Input: part model. Units: mm. Frame: model coordinates. Face numbers are marked on the shaded views. Round coordinates to 2 decimals unless told otherwise and drop trailing zeros. Order: outer loops, then holes, each group sorted by start corner. A loop starts at its lowest first (then second) coordinate and runs counter-clockwise, first axis right, second up. Notation, with made-up numbers: (81, 42) -> (128, 42) arc R12 cw to (128, 61) -> close; hole circle Ø10 at (38, -6.5). An arc over 180 degrees is marked (long way). Use a Markdown table: item, result.
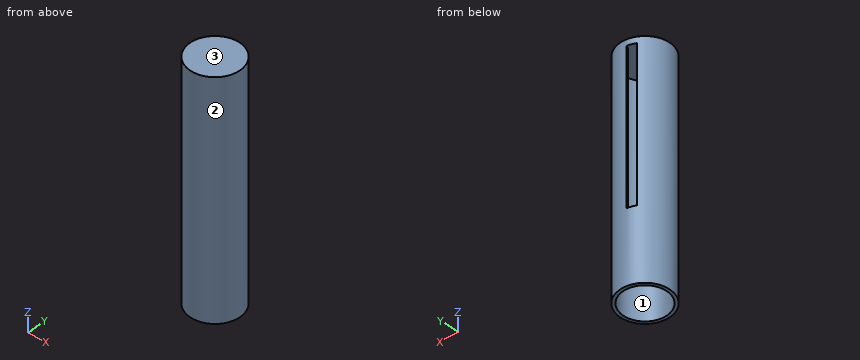
from build123d import *

# Parameters (mm, degrees)
ESQUISSE1_R             = 41
ESQUISSE1_R_2           = 36
BOSS_EXTRU_1_DEPTH      = 370
BOSS_EXTRU_2_DEPTH      = 110
ENL_V_MAT_EXTRU_1_DEPTH = 250
BOSS_EXTRU_3_START      = 10
ESQUISSE3_R             = 41
BOSS_EXTRU_3_DEPTH      = 10


with BuildPart() as part:
    # Esquisse1 → Boss.-Extru.1 (new body)
    with BuildSketch(Plane.XY):
        Circle(ESQUISSE1_R)
        Circle(ESQUISSE1_R_2, mode=Mode.SUBTRACT)
    extrude(amount=-BOSS_EXTRU_1_DEPTH)


with BuildPart() as body_2:
    # Esquisse2 → Boss.-Extru.2 (new body)
    with BuildSketch(Plane.XY):
        Polygon((-20.206852958, 37.47910209), (-6.959206174, 42.006778613), (-0.491096856, 23.081568921), (-13.73874364, 18.553892399), align=None)
    extrude(amount=-BOSS_EXTRU_2_DEPTH)


with BuildPart() as enl_v_mat_extru_1_tool:
    # Esquisse2<2> → Enlèv. mat.-Extru.1 (new body)
    with BuildSketch(Plane.XY):
        Polygon((-20.206852958, 37.47910209), (-6.959206174, 42.006778613), (-0.491096856, 23.081568921), (-13.73874364, 18.553892399), align=None)
    extrude(amount=-ENL_V_MAT_EXTRU_1_DEPTH)


with BuildPart() as part_1:
    add(part.part)

    # Enlèv. mat.-Extru.1: cut by enl_v_mat_extru_1_tool
    add(enl_v_mat_extru_1_tool.part, mode=Mode.SUBTRACT)

    # Esquisse3 → Boss.-Extru.3 (add)
    with BuildSketch(Plane.XY.offset(BOSS_EXTRU_3_START)):
        Circle(ESQUISSE3_R)
    extrude(amount=-BOSS_EXTRU_3_DEPTH)


with BuildPart() as body_2_1:
    add(body_2.part)

    # Enlèv. mat.-Extru.1: cut by enl_v_mat_extru_1_tool
    add(enl_v_mat_extru_1_tool.part, mode=Mode.SUBTRACT)


solid = part_1.part
1) Pin query (flat end, axial travel): pin 1 Ø10 at (y, z) = (-31, -188) entering from -X; pin 2 Ø5 at (y, z) = (31, -294.5) entering from -X; pin 3 Ø2 at (y, z) = (13.5, -200.5) entering from +X. Return the tip coordinate at first contact, or that it passes through.
Results found:
| item | result |
|---|---|
| pin 1 | stops at x = -31.7 |
| pin 2 | stops at x = -29.47 |
| pin 3 | stops at x = 39.05 |
2) Line query: L1, parallel to X at y = 2, z = -215; L2, parallel to Y at x = 0, z = -230; L3, parallel to X at y = -1, z = -330. Output: solid intervals per line, ascending. Write a range as [from, to].
Results found:
| item | result |
|---|---|
| L1 | x = [-40.95, -35.94], [35.94, 40.95] |
| L2 | y = [-41, -36], [36, 41] |
| L3 | x = [-40.99, -35.99], [35.99, 40.99] |
3) Cut plane C-C on z = -289.5. Return loops of the section in (x, y).
Results found:
| item | result |
|---|---|
| outline | circle Ø82 at (0, 0); hole circle Ø72 at (0, 0) |
4) Cut plane D-D on z = -125.5. Return loops of the section in (x, y), and give its area (3 significant figures).
Results found:
| item | result |
|---|---|
| outline | (-19.69, 35.96) arc R41 ccw (long way) to (-6.44, 40.49) -> (-4.8, 35.68) arc R36 cw (long way) to (-18.04, 31.15) -> close |
| area | 1,140 mm² |
5) Cut plane A-A on y = 0. Return loops of the section in (x, z), and give its area (3 significant figures).
Results found:
| item | result |
|---|---|
| outline | (-41, -370) -> (-36, -370) -> (-36, 0) -> (36, 0) -> (36, -370) -> (41, -370) -> (41, 10) -> (-41, 10) -> close |
| area | 4,520 mm² |
6) Pull-direction query (Y, two-part tool) for the marked faces 1, 2 and 3; classes: +Y half, -Y half, draft (parallel to the pull), parting line (faces both ways), or undercut.
Results found:
| item | result |
|---|---|
| face 1 | undercut |
| face 2 | parting line |
| face 3 | draft |
